from build123d import *

# Parameters (mm, degrees)
SKETCH1_W           = 11
SKETCH1_H           = 17
SKETCH1_W_2         = 7
SKETCH1_H_2         = 13
BOSS_EXTRUDE1_DEPTH = 76.2
SKETCH2_W           = 11
SKETCH2_H           = 17
BOSS_EXTRUDE2_DEPTH = 2
SKETCH3_W           = 7
SKETCH3_H           = 11
CUT_EXTRUDE1_DEPTH  = 2
SKETCH4_R           = 19.05
SKETCH4_W           = 11
SKETCH4_H           = 17
BOSS_EXTRUDE3_DEPTH = 3
SKETCH5_R           = 12.7
SKETCH5_W           = 11
SKETCH5_H           = 17
BOSS_EXTRUDE4_DEPTH = 2.54


with BuildPart() as part:
    # Sketch1 → Boss-Extrude1 (new body)
    with BuildSketch(Plane.XY):
        with Locations((3.5, 6.5)):
            Rectangle(SKETCH1_W, SKETCH1_H)
        with Locations((3.5, 6.5)):
            Rectangle(SKETCH1_W_2, SKETCH1_H_2, mode=Mode.SUBTRACT)
    extrude(amount=BOSS_EXTRUDE1_DEPTH)

    # Sketch2 → Boss-Extrude2 (add)
    with BuildSketch(Plane(origin=(0, 0, 0), x_dir=(-1, 0, 0), z_dir=(0, 0, -1))):
        with Locations((-3.5, 6.5)):
            Rectangle(SKETCH2_W, SKETCH2_H)
    extrude(amount=BOSS_EXTRUDE2_DEPTH)

    # Sketch3 → Cut-Extrude1 (cut)
    with BuildSketch(Plane(origin=(0, -2, 0), x_dir=(-1, 0, 0), z_dir=(0, -1, 0))):
        with Locations((-3.5, -5.5)):
            Rectangle(SKETCH3_W, SKETCH3_H)
    extrude(amount=-CUT_EXTRUDE1_DEPTH, mode=Mode.SUBTRACT)

    # Sketch4 → Boss-Extrude3 (add)
    with BuildSketch(Plane.XY.offset(14.986)):
        with Locations((3.5, 6.5)):
            Circle(SKETCH4_R)
        with Locations((3.5, 6.5)):
            Rectangle(SKETCH4_W, SKETCH4_H, mode=Mode.SUBTRACT)
    extrude(amount=BOSS_EXTRUDE3_DEPTH)

    # Sketch5 → Boss-Extrude4 (add)
    with BuildSketch(Plane(origin=(0, 0, 14.986), x_dir=(-1, 0, 0), z_dir=(0, 0, -1))):
        with Locations((-3.5, 6.5)):
            Circle(SKETCH5_R)
        with Locations((-3.5, 6.5)):
            Rectangle(SKETCH5_W, SKETCH5_H, mode=Mode.SUBTRACT)
    extrude(amount=BOSS_EXTRUDE4_DEPTH)


solid = part.part
Verification items for the finished model (mm, model axes). A direction names the side the tool comes from. Round coordinates to 2 decimals unless told otherwise and drop trailing zeros. Write each loop counter-clockwise with the first axis right and the second up, starting at its lowest first coordinate (ties: lowest second). Pieces come first, ordered by that corner, then holes.
(1) Access from +Z, -Z, +X, -X, +Y, -Y to the whole of each face (thin tool, end or side, straight path). Record for faces 1 (the flat face through (3, 0, 43)), 2 (the flat face through (-2, 6, 5)), 3 (the flat face through (-2, 6, 48)), 4 (the flat face through (4, 15, 5)).
Returned:
face 1: +Z
face 2: -Z, -X, +Y, -Y
face 3: +Z, -X, +Y, -Y
face 4: -Z, +X, -X, +Y
(2) Section check B-B (x = 3.5). Enter the section's corners in (y, z).
Returned:
outline: (-12.55, 14.99) - (-6.2, 14.99) - (-6.2, 12.45) - (-2, 12.45) - (-2, 11) - (0, 11) - (0, 76.2) - (-2, 76.2) - (-2, 17.99) - (-12.55, 17.99) - close; (-2, -2) - (15, -2) - (15, 12.45) - (19.2, 12.45) - (19.2, 14.99) - (25.55, 14.99) - (25.55, 17.99) - (15, 17.99) - (15, 76.2) - (13, 76.2) - (13, 0) - (-2, 0) - close
(3) Material ranges on line 1 (X direction, y = 7, z = 59.5); line 2 (Z direction, x = -5, y = 17); line 3 (Z direction, x = -8, y = 5), recorded low to high.
Returned:
line 1: x = -2 to 0, 7 to 9
line 2: z = 14.99 to 17.99
line 3: z = 12.45 to 17.99
(4) Mould release check, pull along X, two halves, no side actions. Record for faces 5 (the flat face through (9, 6, 5)), 6 (the flat face through (0, 5, 38)), 7 (the flat face through (4, 15, 48)): pulls with the +X half, pulls with the -X half, needs draft (parallel to the pull), parting line crosses it, or undercut.
Returned:
face 5: pulls with the +X half
face 6: undercut
face 7: needs draft
(5) Section check A-A (z = 64). Enter the section's corners in (x, y), plus the area to 3 significant figures.
Returned:
outline: (-2, -2) - (9, -2) - (9, 15) - (-2, 15) - close; hole (0, 0) - (7, 0) - (7, 13) - (0, 13) - close
area: 96.0 mm2
(6) Section check D-D (x = -4). Enter the section's corners in (y, z).
Returned:
outline: (-11.01, 14.99) - (-3.75, 14.99) - (-3.75, 12.45) - (16.75, 12.45) - (16.75, 14.99) - (24.01, 14.99) - (24.01, 17.99) - (-11.01, 17.99) - close
(7) Depth check by flat-ended pin: pin 1 Ø8 at (x, y) = (13.5, 5) entering from -Z; pin 2 Ø4.5 at (y, z) = (3, 2.5) entering from +X; pin 3 Ø12 at (x, z) = (6, 3.5) entering from -Y; pin 4 Ø11.5 at (x, y) = (1.5, 3.5) entering from +Z. Enter the tip coordinate at first touch or a pass-through.
Returned:
pin 1: stops at z = 12.45
pin 2: stops at x = 9
pin 3: stops at y = -2
pin 4: stops at z = 76.2
(8) Section check C-C (y = 6.5). Enter the section's corners in (x, z).
Returned:
outline: (-15.55, 14.99) - (-9.2, 14.99) - (-9.2, 12.45) - (-2, 12.45) - (-2, -2) - (9, -2) - (9, 12.45) - (16.2, 12.45) - (16.2, 14.99) - (22.55, 14.99) - (22.55, 17.99) - (9, 17.99) - (9, 76.2) - (7, 76.2) - (7, 0) - (0, 0) - (0, 76.2) - (-2, 76.2) - (-2, 17.99) - (-15.55, 17.99) - close
